Study the drawing (mm; zero at the part's minimum x, y, z) and answer. Coordinates: 2 decimals unless noted, no trailing zeros. Order: outer loops, then holes, each group sorted by start corner. A loop starts at its lowest first (then second) coordinate and runs counter-clockwise, first axis right, second up. Notation, with made-up numbers: M 79,0.25 L 102,0.25 A32 ccw 102,39.25 Z; hole C 51,32 d6. An arc over 180 degrees is marked long. Put each result on its own line as item: value.
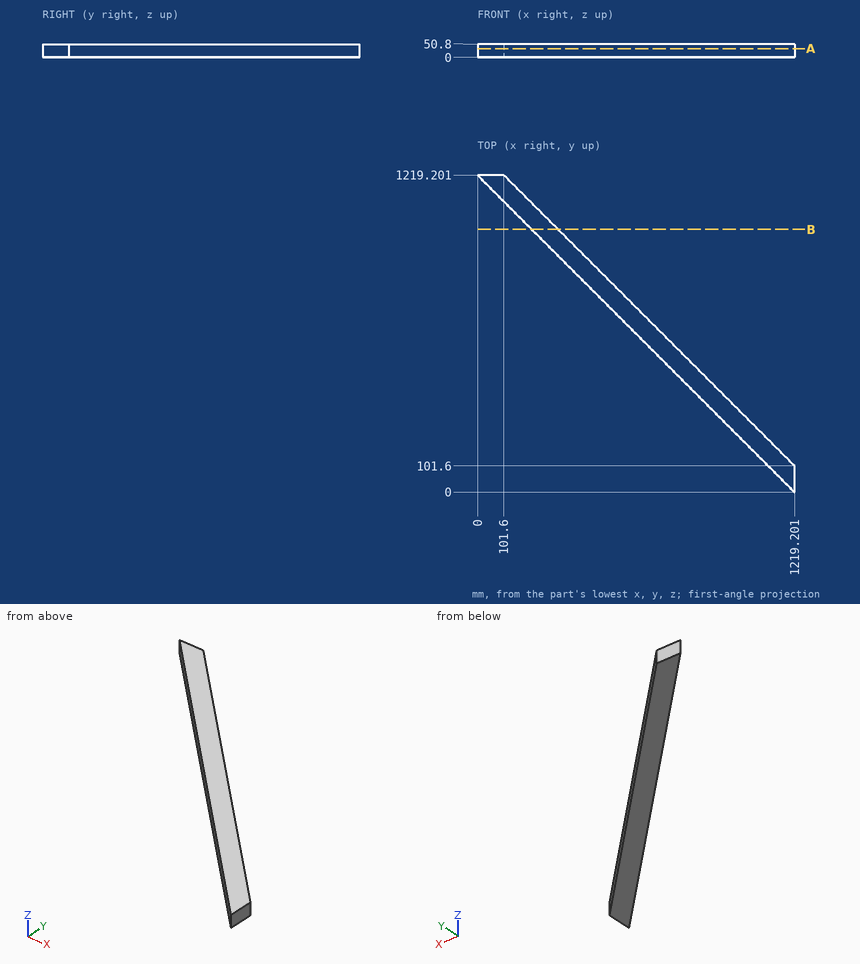
Q1. Find section B-B on y = 1010.5. Write down the section's boundary in (x, z).
Answers below:
outline: M 208.7,0 L 310.3,0 L 310.3,50.8 L 208.7,50.8 Z
Q2. Find section A-A on z = 33. Write down the section's boundary in (x, y).
Answers below:
outline: M 0,1219.2 L 1219.2,0 L 1219.2,101.6 L 101.6,1219.2 Z
Q3. Given pin 1 (1.5 mm diameter, centred on y = 649.5, z = 13, fed in from -X); pin 2 (1 mm diameter, centred on x = 974, z = 15.5, fed in from -Y); pin 3 (1 mm diameter, centred on x = 1055, z = 26, fed in from -Y), each flat-ended and moving along its own axis, determine where each tip first touches the part or whether it passes through.
Answers below:
pin 1: stops at x = 568.95
pin 2: stops at y = 244.7
pin 3: stops at y = 163.7
Q4. Consider line 1 along X through (y, z) = (344, 42.5); line 2 along Y through (x, z) = (560, 32); line 3 along X through (y, z) = (436.5, 30). Determine where each line is inside the solid, lowest interval first.
Answers below:
line 1: x = 875.2 to 976.8
line 2: y = 659.2 to 760.8
line 3: x = 782.7 to 884.3
